Input: dimensioned drawing with shaded views. Units: mm. Origin: part minimum x, y, z. Coordinates: 2 decimals unless noted, no trailing zeros. Loops run counter-clockwise (first coordinate to the right, second up) from the corner with the lowest first, then second, coordinate; pieces in that order, holes last.
Item 1: Section C-C on x = 36.5. Return loops of the section in (y, z), and give its area (3 significant figures).
Item 2: Ray query, line 1 along Z through (x, y) = (5.5, 0.7); line 2 along Z through (x, y) = (35.5, 0.2); line 3 along X through (y, z) = (0.75, 52.5). Return the intervals inside material, ascending.
Item 3: Section B-B on z = 54. Return loops of the section in (x, y).
Item 4: Section A-A on x = 21. Return loops of the section in (y, z).
Item 5: Section D-D on y = 1.1. Return loops of the section in (x, z), and give its area (3 significant figures).
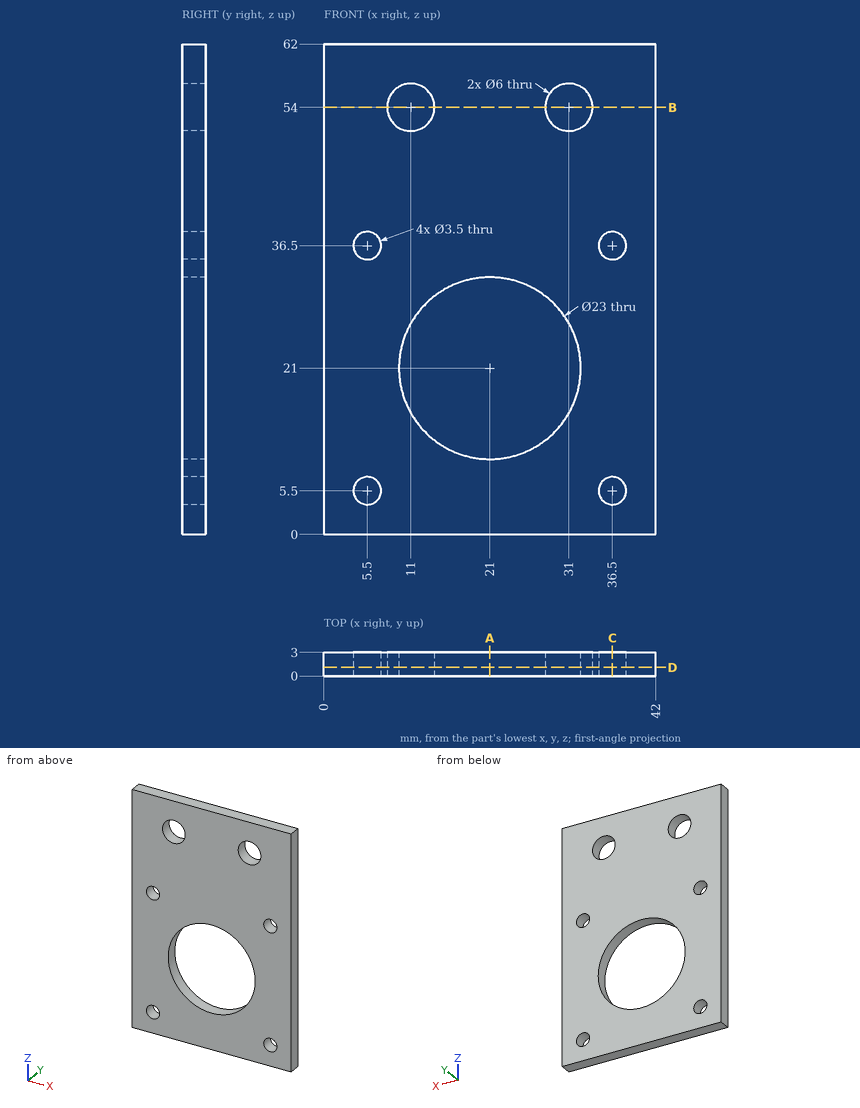
Results found:
1. outline: (0, 0) - (3, 0) - (3, 3.75) - (0, 3.75) - close; (0, 7.25) - (3, 7.25) - (3, 34.75) - (0, 34.75) - close; (0, 38.25) - (3, 38.25) - (3, 62) - (0, 62) - close
1. area: 165 mm2
2. line 1: z = 0 to 3.75, 7.25 to 34.75, 38.25 to 62
2. line 2: z = 0 to 4.06, 6.94 to 35.06, 37.94 to 62
2. line 3: x = 0 to 8.4, 13.6 to 28.4, 33.6 to 42
3. outline: (0, 0) - (8, 0) - (8, 3) - (0, 3) - close; (14, 0) - (28, 0) - (28, 3) - (14, 3) - close; (34, 0) - (42, 0) - (42, 3) - (34, 3) - close
4. outline: (0, 0) - (3, 0) - (3, 9.5) - (0, 9.5) - close; (0, 32.5) - (3, 32.5) - (3, 62) - (0, 62) - close
5. outline: (0, 0) - (42, 0) - (42, 62) - (0, 62) - close; hole circle Ø3.5 at (5.5, 5.5); hole circle Ø3.5 at (5.5, 36.5); hole circle Ø6 at (11, 54); hole circle Ø23 at (21, 21); hole circle Ø6 at (31, 54); hole circle Ø3.5 at (36.5, 5.5); hole circle Ø3.5 at (36.5, 36.5)
5. area: 2,090 mm2
